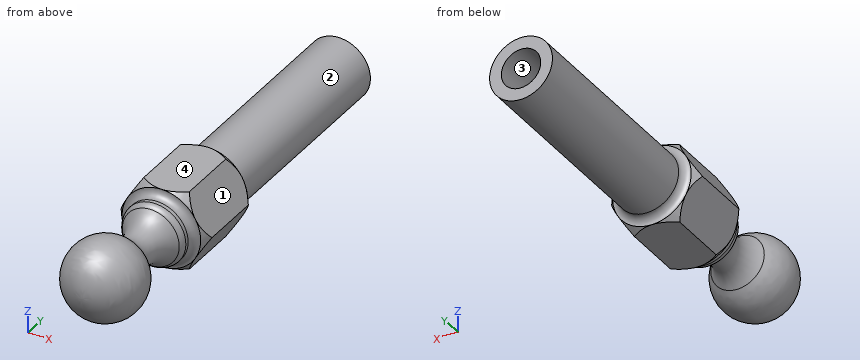
Autodesk Inventor part; units mm, degrees
ref_plane "Work Plane1" through (0, 11, 0) normal (0, 1, 0) x (1, 0, 0)
ref_plane "YZ Plane" through (0, 0, 0) normal (1, 0, 0) x (0, 1, 0)
ref_plane "XZ Plane" through (0, 0, 0) normal (0, 1, 0) x (-1, 0, 0)
sketch "Sketch1" plane through (0, 0, 0) normal (1, 0, 0) x (0, 1, 0)
  arc A0 (-2.5, 0) -> (1.8333, -1.6997) centre (0, 0) ccw
  line L0 (5.254, -2) -> (25, -2)
  line L1 (25, -2) -> (25, -1.25)
  arc A1 (4.8632, -1.8119) -> (1.8333, -1.6997) centre (3.3, -3.0594) ccw
  arc A2 (4.8632, -1.8119) -> (5.254, -2) centre (5.254, -1.5) ccw
  line L2 (25, -1.25) -> (5, -1.25)
  line L3 (5, -1.25) -> (5, 0)
  line L4 (5, 0) -> (-2.5, 0)
  point P0 (4.9964, -2)
  dimension "d0" = 5
  dimension "d2" = 3.3
  dimension "d3" = 4
  dimension "d4" = 25
  dimension "d6" = 0.5
  dimension "d8" = 20
  dimension "d9" = 0.75
  dimension "d10" = 19.746
  dimension "d11" = 5
revolve "Revolution1" add sketch "Sketch1" angle 360 about axis through (0, 5, 0) along (0, -1, 0)
thread "Thread1"
ref_plane "Work Plane1" through (0, 11, 0) normal (0, 1, 0) x (1, 0, 0)
sketch "Sketch2" plane through (0, 11, 0) normal (0, 1, 0) x (1, 0, 0)
  line L0 (1.4434, 2.5) -> (2.8868, 0)
  line L1 (2.8868, 0) -> (1.4434, -2.5)
  line L2 (1.4434, -2.5) -> (-1.4434, -2.5)
  line L3 (-1.4434, -2.5) -> (-2.8868, 0)
  line L4 (-2.8868, 0) -> (-1.4434, 2.5)
  line L5 (-1.4434, 2.5) -> (1.4434, 2.5)
  circle A0 centre (0, 0) radius 1.25
  point P0 (0, 0)
  point P1 (0, 0)
  dimension "d16" = 5
extrude "Extrusion1" add sketch "Sketch2" against normal blind 5
sketch "Sketch3" plane through (0, 11, 0) normal (0, 1, 0) x (1, 0, 0)
  circle A0 centre (0, 0) radius 2.5
  line L0 (-2.8868, 0) -> (-1.4434, 2.5)
extrude "Extrusion2" cut sketch "Sketch3" against normal blind 40 draft 35 and the other way blind 40 keep common part
sketch "Sketch4" plane through (0, 6, 0) normal (0, -1, 0) x (1, 0, 0)
  arc A0 (2.1651, 1.25) -> (0, 2.5) centre (0, 0) ccw
  circle A1 centre (0, 0) radius 2.5
  point P0 (0, 0)
extrude "Extrusion3" cut sketch "Sketch4" against normal blind 40 draft 35 and the other way blind 40 keep common part
fillet "Fillet1" radius 0.5 2 edges at (0, 11, 2) (0, 6, 2)
properties part number "Component 41(Push Rod Base)"
The listing builds one solid part. Answer for the finished solid, in the listing's coordinates (mm). Face numbers are marked on the shaded views. Round coordinates to 2 decimals unless told otherwise and drop trailing zeros. Write each loop counter-clockwise with the first axis right and the second up, starting at its lowest first coordinate (ties: lowest second). Pieces come first, ordered by that corner, then holes. Notation, with made-up numbers: (16.5, 11) -> (46.5, 11) arc R29 cw to (46.5, 48) -> close; hole circle Ø8 at (-24.75, 42.5). An arc over 180 degrees is marked (long way). Use CSV: the item, a comma, the result in double quotes. Start each with the question number.
(1) Each of these flat-tipped pins is pushed along its axis until it touches: pin 1 (1.5 mm diameter, centred on y = 14.5, z = -0.5, fed in from -X); pin 2 (1.5 mm diameter, centred on x = 1.5, z = 0, fed in from -Y); pin 3 (2 mm diameter, centred on x = -1.5, y = 14.5, fed in from -Z). Where does it stop, or does it pass through?
(2) Consider L1, parallel to X at y = 14.5, z = 0; L2, parallel to Y at x = 1.9, z = -0.85; L3, parallel to Y at x = 0.2, z = 2.05. Determine where each line is inside the solid, lowest interval first. Write a range as from..to.
(3) Section A-A on y = 10 is taken. Give the vertices of the cut face in (x, z), then the cut area to 3 significant figures.
(4) The mould has two halves that part along X. Classify the marked faces 1, 2, 3 and 4: released by +X, released by -X, zero draft, split by the parting line, or undercut.
A:
1,pin 1,"stops at x = -2"
1,pin 2,"stops at y = -2.38"
1,pin 3,"stops at z = -1.94"
2,L1,"x = -2..-1.25, 1.25..2"
2,L2,"y = -1.38..1.38, 5.77..11.23"
2,L3,"y = -1.42..1.42, 5.74..11.26"
3,outline,"(-2.89, 0) -> (-1.44, -2.5) -> (1.44, -2.5) -> (2.89, 0) -> (1.44, 2.5) -> (-1.44, 2.5) -> close; hole circle Ø2.5 at (0, 0)"
3,area,"16.7 mm²"
4,face 1,"released by +X"
4,face 2,"split by the parting line"
4,face 3,"undercut"
4,face 4,"zero draft"
